from build123d import *

# Parameters (mm, degrees)
SKETCH1_R                  = 2.25
BASE_FLANGE1_DEPTH         = 1.5875
SKETCHED_START             = -44.45
SKETCHED_BEND1_OUTLINE_W   = 127
SKETCHED_BEND1_OUTLINE_H   = 1.5875
SKETCHED_BEND1_DEPTH       = 27.452834079
SKETCHED_START_2           = -16.777817363
SKETCHED_BEND1_2_OUTLINE_W = 127
SKETCHED_BEND1_2_OUTLINE_H = 28.109665921
SKETCHED_BEND1_2_OUTLINE_R = 2.25
SKETCHED_BEND1_2_DEPTH     = 1.368151442
SKETCHED_START_3           = -16.997165921
SKETCHED_BEND1_3_OUTLINE_W = 127
SKETCHED_BEND1_3_OUTLINE_H = 28.109665921
SKETCHED_BEND1_3_OUTLINE_R = 2.25
SKETCHED_BEND1_3_DEPTH     = 2.3241
SKETCHED_START_4           = -64
SKETCHED_BEND1_4_DEPTH     = 128


with BuildPart() as part:
    # Base-Flange1: sheet metal written as solids
    # Sketch1 → Base-Flange1 (new body)
    with BuildSketch(Plane.XY):
        Polygon((63.5, -12.7), (63.5, 12.7), (-63.5, 12.7), (-63.5, -12.7), (-63.5, -19.05), (-63.5, -44.45), (63.5, -44.45), (63.5, -19.05), align=None)
        with Locations((-57.15, 0)):
            Circle(SKETCH1_R, mode=Mode.SUBTRACT)
        with Locations((-19.05, 0)):
            Circle(SKETCH1_R, mode=Mode.SUBTRACT)
        with Locations((19.05, 0)):
            Circle(SKETCH1_R, mode=Mode.SUBTRACT)
        with Locations((57.15, 0)):
            Circle(SKETCH1_R, mode=Mode.SUBTRACT)
        with Locations(Location((57.15, -31.75, 0), (0, 0, 180))):
            Circle(SKETCH1_R, mode=Mode.SUBTRACT)
        with Locations(Location((19.05, -31.75, 0), (0, 0, 180))):
            Circle(SKETCH1_R, mode=Mode.SUBTRACT)
        with Locations(Location((-19.05, -31.75, 0), (0, 0, 180))):
            Circle(SKETCH1_R, mode=Mode.SUBTRACT)
        with Locations(Location((-57.15, -31.75, 0), (0, 0, 180))):
            Circle(SKETCH1_R, mode=Mode.SUBTRACT)
    extrude(amount=-BASE_FLANGE1_DEPTH)

    # Sketched Bend1: read off the stored shape, not the designer's step
    # Sketched Bend1 outline → Sketched Bend1 (cut)
    with BuildSketch(Plane(origin=(0, 0, 0), x_dir=(1, 0, 0), z_dir=(0, 1, 0)).offset(SKETCHED_START)):
        with Locations((0, 0.79375)):
            Rectangle(SKETCHED_BEND1_OUTLINE_W, SKETCHED_BEND1_OUTLINE_H)
    extrude(amount=SKETCHED_BEND1_DEPTH, mode=Mode.SUBTRACT)

    # Sketched Bend1 2 outline → Sketched Bend1 2 (add)
    with BuildSketch(Plane(origin=(0, 0, 0), x_dir=(1, 0, 0), z_dir=(0, 1, 0)).offset(SKETCHED_START_2)):
        with Locations((0, 15.642332961)):
            Rectangle(SKETCHED_BEND1_2_OUTLINE_W, SKETCHED_BEND1_2_OUTLINE_H)
        with Locations((-57.15, 16.997165921)):
            Circle(SKETCHED_BEND1_2_OUTLINE_R, mode=Mode.SUBTRACT)
        with Locations((-19.05, 16.997165921)):
            Circle(SKETCHED_BEND1_2_OUTLINE_R, mode=Mode.SUBTRACT)
        with Locations((19.05, 16.997165921)):
            Circle(SKETCHED_BEND1_2_OUTLINE_R, mode=Mode.SUBTRACT)
        with Locations((57.15, 16.997165921)):
            Circle(SKETCHED_BEND1_2_OUTLINE_R, mode=Mode.SUBTRACT)
    extrude(amount=SKETCHED_BEND1_2_DEPTH)

    # Sketched Bend1 3 outline → Sketched Bend1 3 (add)
    with BuildSketch(Plane(origin=(0, 0, 0), x_dir=(1, 0, 0), z_dir=(0, 1, 0)).offset(SKETCHED_START_3)):
        with Locations((0, 15.642332961)):
            Rectangle(SKETCHED_BEND1_3_OUTLINE_W, SKETCHED_BEND1_3_OUTLINE_H)
        with Locations((-57.15, 16.997165921)):
            Circle(SKETCHED_BEND1_3_OUTLINE_R, mode=Mode.SUBTRACT)
        with Locations((-19.05, 16.997165921)):
            Circle(SKETCHED_BEND1_3_OUTLINE_R, mode=Mode.SUBTRACT)
        with Locations((19.05, 16.997165921)):
            Circle(SKETCHED_BEND1_3_OUTLINE_R, mode=Mode.SUBTRACT)
        with Locations((57.15, 16.997165921)):
            Circle(SKETCHED_BEND1_3_OUTLINE_R, mode=Mode.SUBTRACT)
    extrude(amount=SKETCHED_BEND1_3_DEPTH)

    # Sketched Bend1 4 outline → Sketched Bend1 4 (cut)
    with BuildSketch(Plane.YZ.offset(SKETCHED_START_4)):
        with BuildLine():
            ThreePointArc((-14.673065921, -1.5875), (-15.193920776, -1.803245145), (-15.409665921, -2.3241))
            Line((-15.409665921, -2.3241), (-15.409665921, -29.697165921))
            Line((-15.409665921, -29.697165921), (-14.673065921, -29.697165921))
            Line((-14.673065921, -29.697165921), (-14.673065921, -1.5875))
        make_face()
        with BuildLine():
            Line((-16.997165921, 0), (-16.997165921, -2.3241))
            ThreePointArc((-16.997165921, -2.3241), (-16.316452791, -0.68071313), (-14.673065921, 0))
            Line((-14.673065921, 0), (-16.997165921, 0))
        make_face()
    extrude(amount=SKETCHED_BEND1_4_DEPTH, mode=Mode.SUBTRACT)


solid = part.part
Can you work these out from the model? Positions are in its coordinate system, mm. Coordinates: 2 decimals unless noted, no trailing zeros. Loops run counter-clockwise (first coordinate to the right, second up) from the corner with the lowest first, then second, coordinate; pieces in that order, holes last. Notation, with made-up numbers: M 0.25,36 L 32.25,36 A21 cw 32.25,59 Z; hole C 31.5,-40 d5. An arc over 180 degrees is marked long. Return JSON: item names as keys, results as strings. Group by question number.
Item 1: Imagine slicing it at C-C (z = -5.5). Please give me the cut outline in (x, y).
Item 2: Thinking about a two-plate mould opening in Y: for faces 1 (the cylindrical face through (-0.889, -16.334, -0.699)), 2 (the flat face through (-1, -1, -1.588)), 3 (the flat face through (-1, -15.41, -16)), 4 (the cylindrical face through (-20.71, 1.52, -0.78)), which applies, released by +Y, released by -Y, zero draft, split by the parting line, or undercut?
Item 3: I'm going to push flat-ended pins straight in: pin 1 Ø8 at (x, z) = (-21, -21.5) entering from +Y; pin 2 Ø12 at (x, y) = (48.5, -5) entering from -Z. Where does each tip first touch, or does it pass through?
Item 4: Imagine slicing it at A-A (x = 19.05). Please give me the cut outline in (y, z).
Item 5: Imagine slicing it at B-B (y = 0). Please give me the cut outline in (x, z), and give its area (3 significant figures).
Item 6: If I drill on L1, parallel to Z at x = 9.5, y = 1; L2, parallel to Y at x = 35, z = -15.5; L3, parallel to Y at x = 57.15, z = -0.55, over which ranges is the centre line in solid material (lowest first)? Write a range as from..to.
Verdict:
{
 "1": {"outline": "M -63.5,-17 L 63.5,-17 L 63.5,-15.41 L -63.5,-15.41 Z"},
 "2": {"face 1": "released by -Y", "face 2": "zero draft", "face 3": "released by +Y", "face 4": "undercut"},
 "3": {"pin 1": "stops at y = -15.41", "pin 2": "stops at z = -1.59"},
 "4": {"outline": "M -17,-29.7 L -15.41,-29.7 L -15.41,-19.25 L -17,-19.25 Z; M -17,-14.75 L -15.41,-14.75 L -15.41,-2.32 A0.74 cw -14.67,-1.59 L -2.25,-1.59 L -2.25,0 L -14.67,0 A2.32 ccw -17,-2.32 Z; M 2.25,-1.59 L 12.7,-1.59 L 12.7,0 L 2.25,0 Z"},
 "5": {"outline": "M -63.5,-1.59 L -59.4,-1.59 L -59.4,0 L -63.5,0 Z; M -54.9,-1.59 L -21.3,-1.59 L -21.3,0 L -54.9,0 Z; M -16.8,-1.59 L 16.8,-1.59 L 16.8,0 L -16.8,0 Z; M 21.3,-1.59 L 54.9,-1.59 L 54.9,0 L 21.3,0 Z; M 59.4,-1.59 L 63.5,-1.59 L 63.5,0 L 59.4,0 Z", "area": "173 mm^2"},
 "6": {"L1": "z = -1.59..0", "L2": "y = -17..-15.41", "L3": "y = -16.17..-2.25, 2.25..12.7"}
}
